For this review, take the finished solid that the model builds, in its own axes (mm). Face numbers are marked on the shaded views. A direction names the side the tool comes from. Give positions to 0.01 mm unless a question says otherwise; leave off trailing zeros. Order: outer loops, then holes, each group sorted by start corner. A loop starts at its lowest first (then second) coordinate and runs counter-clockwise, first axis right, second up. Notation, with made-up numbers: (57, 44.25) - (100, 44.25) arc R27 cw to (100, 76.25) - close; hole circle Ø8 at (-10, -22.75). An arc over 180 degrees is marked (long way). Answer as a JSON object with one key per item and string values. Group by question number.
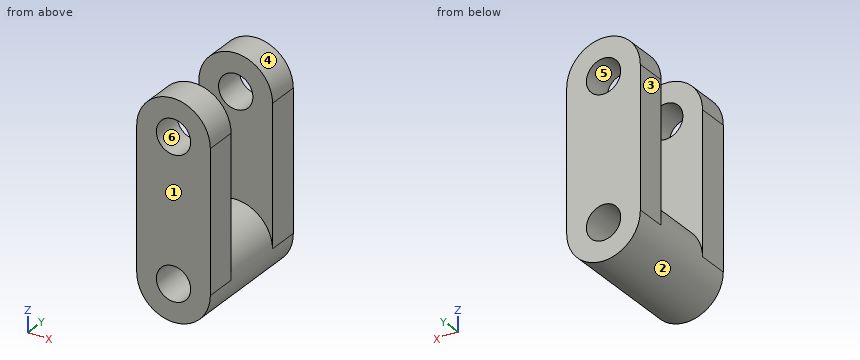
from build123d import *

# Parameters (mm, degrees)
F0_R     = 13.797693
F1_DEPTH = 25.4
F2_R     = 29.61701
F2_R_2   = 13.794222
F3_DEPTH = 101.6
F4_R     = 13.798954
F5_DEPTH = 25.4


with BuildPart() as f1:
    # F0 (on Front) → F1 (new body)
    with BuildSketch(Plane.XZ):
        with BuildLine():
            ThreePointArc((-29.61701, -56.529284), (0, -26.912274), (29.61701, -56.529284))
            Line((29.61701, -56.529284), (29.61701, 56.529284))
            ThreePointArc((29.61701, 56.529284), (0, 86.146293), (-29.61701, 56.529284))
            Line((-29.61701, 56.529284), (-29.61701, -56.529284))
        make_face()
        with Locations((0, 56.529284)):
            Circle(F0_R, mode=Mode.SUBTRACT)
    extrude(amount=-F1_DEPTH)

    # F2 (on face) → F3 (join)
    with BuildSketch(Plane.XZ):
        with Locations((0, -56.529284)):
            Circle(F2_R)
        with Locations((0, -56.529284)):
            Circle(F2_R_2, mode=Mode.SUBTRACT)
    extrude(amount=-F3_DEPTH)

    # F4 (on face) → F5 (join)
    with BuildSketch(Plane(origin=(0, 101.6, 0), x_dir=(-1, 0, 0), z_dir=(0, 1, 0))):
        with BuildLine():
            ThreePointArc((-29.612104, -55.99023), (0, -26.912274), (29.612104, -55.99023))
            Line((29.612104, -55.99023), (29.612104, 55.99023))
            ThreePointArc((29.612104, 55.99023), (0, 85.602334), (-29.612104, 55.99023))
            Line((-29.612104, 55.99023), (-29.612104, -55.99023))
        make_face()
        with Locations((0, 55.99023)):
            Circle(F4_R, mode=Mode.SUBTRACT)
    extrude(amount=-F5_DEPTH)


solid = f1.part
1) Consider section C-C (y = 7). Give the boundary of the cut face in (x, z).
2) Mouldability with a two-part tool opening along Y and no side actions: class the marked faces 1, 2 and 3 as released by +Y, released by -Y, zero draft, split by the parting line, or undercut.
3) Consider section B-B (x = 0). Give the boundary of the cut face in (y, z), plus the area to 3 significant figures.
4) Consider section A-A (z = 6.5). Give the boundary of the cut face in (x, y), plus the area to 3 significant figures.
5) For line 1 (Z direction, x = 0, y = 9.5); line 2 (Z direction, x = 0, y = 87); line 3 (Z direction, x = 0, y = 66), list the stretches that pass through material, from the lowest coordinate up.
6) For the marked faces 4, 5 and 6, list the 3-axis set-ups (+Z, -Z, +X, -X, +Y, -Y) from which the entire face can be reached by the end or side of a thin tool; tool diameter is ignored.
7) For pin 1 (12 mm diameter, centred on y = 73, z = 24.5, fed in from +X); pin 2 (8 mm diameter, centred on x = 10.5, z = -59.5, fed in from -Y); pin 3 (7.5 mm diameter, centred on y = 90.5, z = 23.5, fed in from -X); pin 4 (1 mm diameter, centred on y = 64.5, z = -43.5, fed in from +X), all flat-tipped, find the tip position at first contact; note any pin that passes through.
8) Consider section D-D (z = 65.5). Give the boundary of the cut face in (x, y).
Result set:
{
 "1": {"outline": "(-29.62, -56.53) arc R29.62 ccw to (29.62, -56.53) - (29.62, 56.53) arc R29.62 ccw to (-29.62, 56.53) - close; hole circle Ø27.6 at (0, 56.53); hole circle Ø27.59 at (0, -56.53)"},
 "2": {"face 1": "released by -Y", "face 2": "undercut", "face 3": "zero draft"},
 "3": {"outline": "(0, -86.15) - (101.6, -86.15) - (101.6, -70.32) - (0, -70.32) - close; (0, -42.74) - (101.6, -42.74) - (101.6, 42.19) - (76.2, 42.19) - (76.2, -26.91) - (25.4, -26.91) - (25.4, 42.73) - (0, 42.73) - close; (0, 70.33) - (25.4, 70.33) - (25.4, 86.15) - (0, 86.15) - close; (76.2, 69.79) - (101.6, 69.79) - (101.6, 85.6) - (76.2, 85.6) - close", "area": "7,540 mm2"},
 "4": {"outline": "(-29.62, 0) - (29.62, 0) - (29.62, 25.4) - (-29.62, 25.4) - close; (-29.61, 76.2) - (29.61, 76.2) - (29.61, 101.6) - (-29.61, 101.6) - close", "area": "3,010 mm2"},
 "5": {"line 1": "z = -86.15 to -70.32, -42.74 to 42.73, 70.33 to 86.15", "line 2": "z = -86.15 to -70.32, -42.74 to 42.19, 69.79 to 85.6", "line 3": "z = -86.15 to -70.32, -42.74 to -26.91"},
 "6": {"face 4": "+Z, +Y", "face 5": "+Y", "face 6": "-Y"},
 "7": {"pin 1": "stops at x = 29.61", "pin 2": "stops at y = 0", "pin 3": "stops at x = -29.61", "pin 4": "stops at x = 26.84"},
 "8": {"outline": "(-28.23, 0) - (-10.48, 0) - (-10.48, 25.4) - (-28.23, 25.4) - close; (-28.04, 76.2) - (-10, 76.2) - (-10, 101.6) - (-28.04, 101.6) - close; (10, 76.2) - (28.04, 76.2) - (28.04, 101.6) - (10, 101.6) - close; (10.48, 0) - (28.23, 0) - (28.23, 25.4) - (10.48, 25.4) - close"}
}
